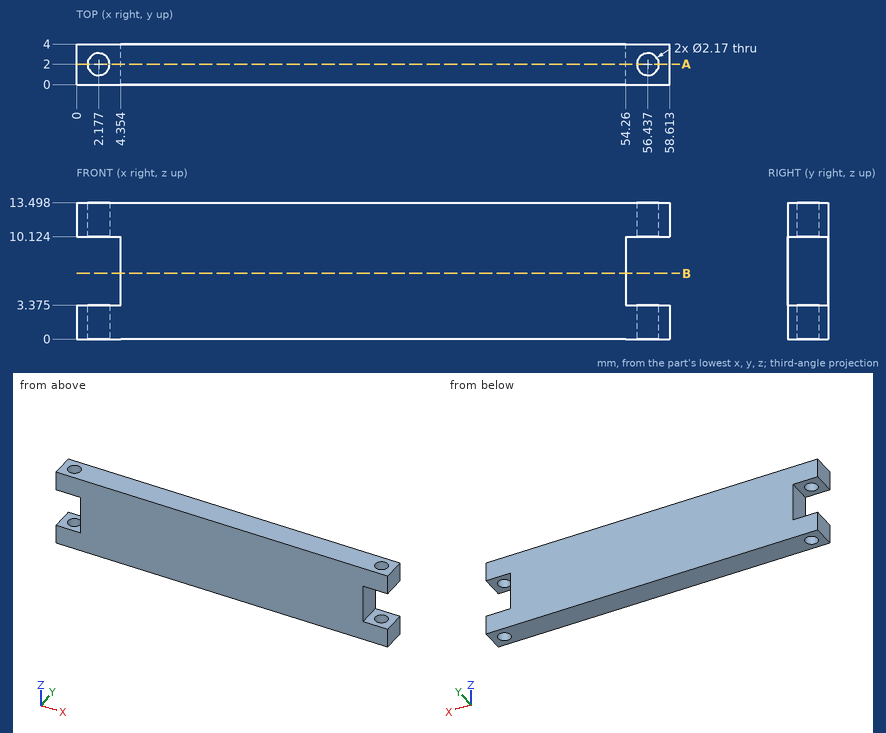
Source: three-view drawing plus pictorial views. Frame: mm from the lowest corner of the part. Give positions to 0.01 mm unless a question says otherwise; leave off trailing zeros. Loops run counter-clockwise (first coordinate to the right, second up) from the corner with the lowest first, then second, coordinate; pieces in that order, holes last. Notation, with made-up numbers: M -17,31 L 23,31 A31 ccw 23,57 Z; hole C -21,52.25 d11. An arc over 180 degrees is marked long. Put each result on its own line as item: value.
Q1. Section A-A (y = 2). Return the cut outline in (x, z) (1 decimal), and give its area (3 significant figures).
Response values:
outline: M 0,0 L 1.1,0 L 1.1,3.4 L 0,3.4 Z; M 0,10.1 L 1.1,10.1 L 1.1,13.5 L 0,13.5 Z; M 3.3,0 L 55.4,0 L 55.4,3.4 L 54.3,3.4 L 54.3,10.1 L 55.4,10.1 L 55.4,13.5 L 3.3,13.5 L 3.3,10.1 L 4.4,10.1 L 4.4,3.4 L 3.3,3.4 Z; M 57.5,0 L 58.6,0 L 58.6,3.4 L 57.5,3.4 Z; M 57.5,10.1 L 58.6,10.1 L 58.6,13.5 L 57.5,13.5 Z
area: 703 mm²
Q2. Section B-B (z = 6.5). Return the cut outline in (x, y), and give its area (3 significant figures).
Response values:
outline: M 4.35,0 L 54.26,0 L 54.26,4 L 4.35,4 Z
area: 200 mm²
Q3. Line query: probe 1 along Z at (x, y) = (55.5, 1.1) (1 decimal); probe 2 along X at (y, z) = (1.4, 11.5) (1 decimal); probe 3 along X at (y, z) = (2.2, 10.75). Output: solid intervals per line, ascending. Write a range as [from, to].
Response values:
probe 1: z = [0, 3.4], [10.1, 13.5]
probe 2: x = [0, 1.3], [3.1, 55.5], [57.3, 58.6]
probe 3: x = [0, 1.11], [3.24, 55.37], [57.5, 58.61]
Q4. Pin query (flat end, axial travel): P1, Ø1.2, axis at y = 2, z = 7, coming from the +X side; P2, Ø1.3, axis at x = 2.18, y = 2, coming from the -Z side; P3, Ø2, axis at y = 2.5, z = 6, coming from the -X side. Return the tip coordinate at first contact, or that it passes through.
Response values:
P1: stops at x = 54.26
P2: passes through
P3: stops at x = 4.35
